The model under review builds one solid part; all positions refer to its coordinate system, in mm. Give positions to 0.01 mm unless a question says otherwise; leave off trailing zeros. Loops run counter-clockwise (first coordinate to the right, second up) from the corner with the lowest first, then second, coordinate; pieces in that order, holes last. Notation, with made-up numbers: M 24,46.25 L 41,46.25 A26 cw 41,78.25 Z; hole C 3.5,82 d9. An arc over 180 degrees is marked long. One line per item, written item: value. Start each with the question number.
Q1. We need section A-A on x = 56.5. Write out the cut boundary in (y, z).
Q2. We need section B-B on x = -12.5. Write out the cut boundary in (y, z), plus the area to 3 significant figures.
Q3. For pin 1 (1.5 mm diameter, centred on x = 11.5, z = 1, fed in from +Y) (3 decimals); pin 2 (2.5 mm diameter, centred on x = 56.5, y = 9, fed in from +Z), all flat-tipped, find the tip position at first contact; note any pin that passes through.
Q4. To check wall thickness, follow line 1 along Y through (x, z) = (56.5, 1.45); line 2 along Y through (x, z) = (-11, 3.6); line 3 along X through (y, z) = (59, 2.95). State the ranges of each line that lie inside material, in increasing order. Write a range as from..to.
Q5. We need section C-C on y = 62.5. Write out the cut boundary in (x, z), plus the area to 3 significant figures.
Q6. We need section D-D on z = 3.4. Write out the cut boundary in (x, y).
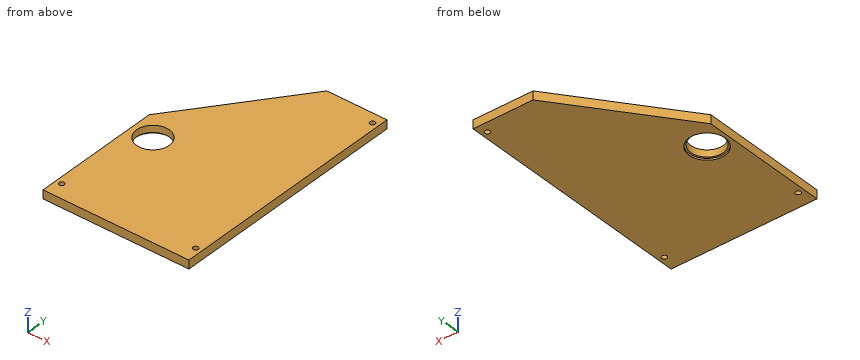
```python
from build123d import *

# Parameters (mm, degrees)
SKETCH1_R           = 1.5
SKETCH1_R_2         = 10.5
BOSS_EXTRUDE1_DEPTH = 5
BOSS_EXTRUDE2_START = 1
SKETCH1_3_R         = 10.5
SKETCH1_3_R_2       = 9.5
BOSS_EXTRUDE2_DEPTH = 4


with BuildPart() as part:
    # Sketch1 → Boss-Extrude1 (new body)
    with BuildSketch(Plane.XY):
        Polygon((-25, 0), (50, 0), (60, 0), (60, 140), (25, 140), (-25, 75), align=None)
        with Locations((-21.5, 9)):
            Circle(SKETCH1_R, mode=Mode.SUBTRACT)
        with Locations((-12.5, 62.5)):
            Circle(SKETCH1_R_2, mode=Mode.SUBTRACT)
        with Locations((56.5, 9)):
            Circle(SKETCH1_R, mode=Mode.SUBTRACT)
        with Locations((56.5, 134)):
            Circle(SKETCH1_R, mode=Mode.SUBTRACT)
    extrude(amount=BOSS_EXTRUDE1_DEPTH)

    # Sketch1<3> → Boss-Extrude2 (add)
    with BuildSketch(Plane.XY.offset(BOSS_EXTRUDE2_START)):
        with Locations((-12.5, 62.5)):
            Circle(SKETCH1_3_R)
        with Locations((-12.5, 62.5)):
            Circle(SKETCH1_3_R_2, mode=Mode.SUBTRACT)
    extrude(amount=BOSS_EXTRUDE2_DEPTH)


solid = part.part
```
Solved:
1. outline: M 0,0 L 7.5,0 L 7.5,5 L 0,5 Z; M 10.5,0 L 132.5,0 L 132.5,5 L 10.5,5 Z; M 135.5,0 L 140,0 L 140,5 L 135.5,5 Z
2. outline: M 0,0 L 52,0 L 52,1 L 53,1 L 53,5 L 0,5 Z; M 72,1 L 73,1 L 73,0 L 91.25,0 L 91.25,5 L 72,5 Z
2. area: 359 mm2
3. pin 1: y = 123.425
3. pin 2: through
4. line 1: 0..7.5, 10.5..132.5, 135.5..140
4. line 2: 0..53.12, 71.88..93.2
4. line 3: -25..-21.33, -3.67..60
5. outline: M -25,0 L -23,0 L -23,1 L -22,1 L -22,5 L -25,5 Z; M -3,1 L -2,1 L -2,0 L 60,0 L 60,5 L -3,5 Z
5. area: 328 mm2
6. outline: M -25,0 L 60,0 L 60,140 L 25,140 L -25,75 Z; hole C -21.5,9 d3; hole C -12.5,62.5 d19; hole C 56.5,9 d3; hole C 56.5,134 d3
